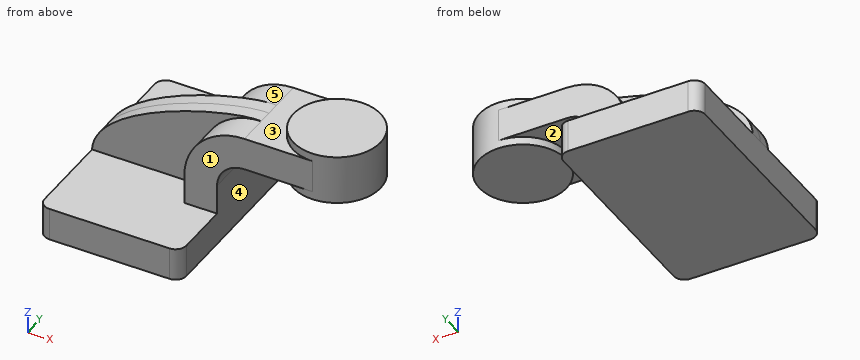
from build123d import *

# Parameters (mm, degrees)
F1_DEPTH = 63.5
F2_DEPTH = 25.4
F3_DEPTH = 7.9375
F5_R     = 6.35


# Not quite as in the source:
# - ends of sketch curves that miss each other by under 0.0002 mm in the source are joined
# - a feature names something its author has since deleted; it is built from what else it names


with BuildPart() as f1:
    # F0 (on Front) → F1 (new body, symmetric)
    with BuildSketch(Plane.XZ):
        Polygon((-41.275, 9.525), (-41.275, -9.525), (41.275, -9.525), (41.275, 9.525), (22.225, 9.525), align=None)
    extrude(amount=F1_DEPTH, both=True)

    # F0 (on Front) → F2 (join, symmetric)
    with BuildSketch(Plane.XZ):
        with BuildLine():
            Line((22.225, 9.525), (41.275, 9.525))
            Line((41.275, 9.525), (41.275, 27.0002))
            ThreePointArc((41.275, 27.0002), (45.9246798487, 38.2255201513), (57.15, 42.8752))
            Line((57.15, 42.8752), (71.4156685244, 42.8752))
            Line((71.4156685244, 42.8752), (71.4156685244, 61.9252))
            Line((71.4156685244, 61.9252), (57.15, 61.9252))
            ThreePointArc((57.15, 61.9252), (32.4542956671, 51.6959043329), (22.225, 27.0002))
            Line((22.225, 27.0002), (22.225, 9.525))
        make_face()
        Polygon((96.8156695652, 61.9252), (71.4156685244, 61.9252), (71.4156685244, 42.8752), (96.8156754971, 42.8752), align=None)
    extrude(amount=F2_DEPTH, both=True)

    # F0 (on Front) → F3 (join, symmetric)
    with BuildSketch(Plane.XZ):
        with BuildLine():
            add(Edge.make_bspline(
                [(-41.275, 9.525), (-40.0072485209, 41.9578626752), (41.6273023615, 64.213483679), (57.15, 61.9252)],
                knots=[0, 0, 0, 0, 111.5045361635, 111.5045361635, 111.5045361635, 111.5045361635], degree=3))
            Line((-41.275, 9.525), (22.225, 9.525))
            Line((22.225, 9.525), (22.225, 27.0002))
            ThreePointArc((22.225, 27.0002), (32.4542956671, 51.6959043329), (57.15, 61.9252))
        make_face()
    extrude(amount=F3_DEPTH, both=True)

    # F0 (on Front) → F4 (revolve)
    with BuildSketch(Plane.XZ):
        Polygon((96.8156685244, 66.675), (96.8156685244, 61.9252), (96.8156685244, 42.8752), (96.8156685244, 38.1), (122.2156685244, 38.1), (122.2156685244, 66.675), align=None)
    revolve(axis=Axis((96.8156685244, 0, 52.3875), (0, 0, 1)))

    # F5
    f5_edges = [f1.edges().sort_by_distance(p)[0] for p in [
        (-41.275, -63.5, 0),
        (-41.275, 63.5, 0),
        (41.275, 63.5, 0),
        (41.275, -63.5, 0),
    ]]
    fillet(f5_edges, radius=F5_R)


solid = f1.part
CAD build for the part. Positions are in the model's coordinates, mm. Face numbers are marked on the shaded views. A direction names the side the tool comes from. Coordinates: 2 decimals unless noted, no trailing zeros. Loops run counter-clockwise (first coordinate to the right, second up) from the corner with the lowest first, then second, coordinate; pieces in that order, holes last. Notation, with made-up numbers: (-32.75, 11.5) - (11.25, 11.5) arc R11 cw to (11.25, 18.5) - close; hole circle Ø2 at (36, 77.5). An arc over 180 degrees is marked (long way). Use one line per item in the form item = value. Start each with the question number.
1) Band-saw the part on D-D (x = 67). Give the cut face in (y, z), and give its area (3 significant figures).
2) Band-saw the part on C-C (x = 90.5). Give the cut face in (y, z) (3 decimals), and give its area (3 significant figures).
3) Band-saw the part on B-B (y = 27.5). Give the cut face in (x, z) (3 decimals), and give its area (3 significant figures).
4) Tool access for the marked faces 1, 2, 3, 4 and 5: list every direction of +Z, -Z, +X, -X, +Y, -Y with a clear straight run to the whole face (end or side of a thin tool).
5) Flat gauge pins, fed straight in: pin 1 (18.5 mm diameter, centred on y = 12.5, z = 2, fed in from +X) (3 decimals); pin 2 (2 mm diameter, centred on x = 36, y = -17, fed in from +Z); pin 3 (8 mm diameter, centred on y = 22, z = 53, fed in from -X) (3 decimals). Where does each tip first touch, or does it go through?
6) Drill centre lines: L1, parallel to Y at x = -1, z = 46; L2, parallel to X at y = 56, z = 5.5 (3 decimals); L3, parallel to X at y = -14.5, z = 10 (3 decimals). Where is each one in solid material? Low to high. Write a range as from..to.
7) Band-saw the part on A-A (z = -3.5). Give the cut face in (x, y) (3 decimals), and give its area (3 significant figures).
Check values:
q1.outline = (-25.4, 42.88) - (25.4, 42.88) - (25.4, 61.93) - (-25.4, 61.93) - close
q1.area = 968 mm2
q2.outline = (-25.4, 42.875) - (-24.602, 42.875) - (-24.602, 38.1) - (24.602, 38.1) - (24.602, 42.875) - (25.4, 42.875) - (25.4, 61.925) - (24.602, 61.925) - (24.602, 66.675) - (-24.602, 66.675) - (-24.602, 61.925) - (-25.4, 61.925) - close
q2.area = 1,440 mm2
q3.outline = (-41.275, -9.525) - (41.275, -9.525) - (41.275, 9.525) - (-41.275, 9.525) - close
q3.area = 1,570 mm2
q4.face_1 = +Z, +X, -X, -Y
q4.face_2 = -Z
q4.face_3 = +Z
q4.face_4 = -Z, +X, +Y, -Y
q4.face_5 = +Z, -X, +Y
q5.pin_1 = 41.275
q5.pin_2 = 55.53
q5.pin_3 = 30.025
q6.L1 = -7.94..7.94
q6.L2 = -41.275..41.275
q6.L3 = 22.225..41.275
q7.outline = (-41.275, -57.15) arc R6.35 ccw to (-34.925, -63.5) - (34.925, -63.5) arc R6.35 ccw to (41.275, -57.15) - (41.275, 57.15) arc R6.35 ccw to (34.925, 63.5) - (-34.925, 63.5) arc R6.35 ccw to (-41.275, 57.15) - close
q7.area = 10,400 mm2
